Check sheet for the modelled part. Datum: model origin and axes. Units: mm. Face numbers are marked on the shaded views. A direction names the side the tool comes from. Round coordinates to 2 decimals unless told otherwise and drop trailing zeros. Write each loop counter-clockwise with the first axis right and the second up, starting at its lowest first coordinate (ties: lowest second). Pieces come first, ordered by that corner, then holes.
Item 1: Material ranges on line 1 along X through (y, z) = (13, 7.25); line 2 along X through (y, z) = (4.25, 4.5); line 3 along Y through (x, z) = (-0.5, -12), recorded low to high.
Item 2: Section check B-B, the plane x = 8. Record the cut outline in (y, z), plus the area to 3 significant figures.
Item 3: Set-up check for the marked faces 1, 2 and 3: record each of +Z, -Z, +X, -X, +Y, -Y from which the full face is reachable in a straight line by a thin tool's end or side.
Item 4: Section check A-A, the plane z = 0. Record the cut outline in (x, y), plus the area to 3 significant figures.
Item 5: Section check D-D, the plane z = -8. Record the cut outline in (x, y).
Item 6: Depth check by flat-ended pin: pin 1 (1.5 mm diameter, centred on y = 7.5, z = -5.5, fed in from +X); pin 2 (1.6 mm diameter, centred on x = 7.5, z = 0, fed in from +Y); pin 3 (2 mm diameter, centred on x = -13, y = 4, fed in from -Z); pin 4 (3 mm diameter, centred on x = -8, z = 0, fed in from -Y). Enter the tip coordinate at first touch or a pass-through.
Item 7: Release check for a two-part mould opening along Z. For the marked faces 4, 5 and 6 record: pulls with the +Z half, pulls with the -Z half, needs draft (parallel to the pull), parting line crosses it, or undercut.
Item 8: Section check C-C, the plane y = 6.75. Record the cut outline in (x, z).
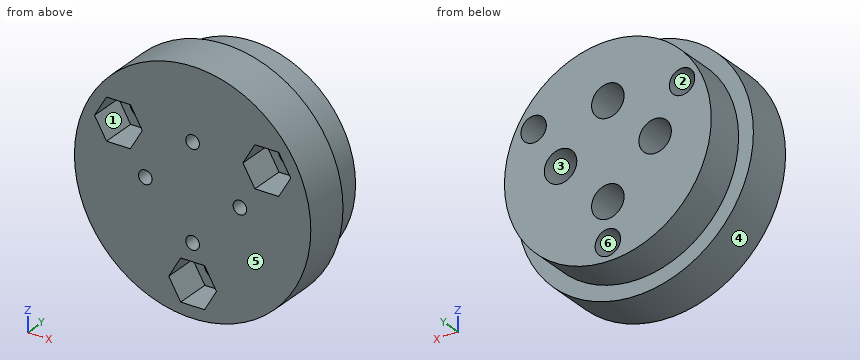
Autodesk Inventor part; units mm, degrees
ref_plane "YZ Plane" through (0, 0, 0) normal (1, 0, 0) x (0, 1, 0)
ref_plane "XZ Plane" through (0, 0, 0) normal (0, 1, 0) x (-1, 0, 0)
ref_plane "XY Plane" through (0, 0, 0) normal (0, 0, 1) x (1, 0, 0)
sketch "Sketch1" plane through (0, 0, 0) normal (0, 1, 0) x (-1, 0, 0)
  circle A0 centre (0, 0) radius 8 construction
  circle A1 centre (8, 0) radius 1 construction
  circle A2 centre (0, -8) radius 1 construction
  circle A3 centre (-8, 0) radius 1 construction
  circle A4 centre (0, 8) radius 1 construction
  circle A5 centre (13, 0) radius 2 construction
  circle A6 centre (-6.5, 11.2583) radius 2 construction
  circle A7 centre (-6.5, -11.2583) radius 2 construction
  line L0 (13, 0) -> (0, 0)
  line L1 (0, 0) -> (0, -5.456)
  circle A8 centre (0, 0) radius 20
  dimension "d0" = 16
  dimension "d1" = 2
  dimension "d2" = 2
  dimension "d3" = 2
  dimension "d4" = 2
  dimension "d5" = 4
  dimension "d8" = 360
  dimension "d10" = 13
  dimension "d11" = 90
  dimension "d12" = 40
extrude "Extrusion1" add sketch "Sketch1" along normal blind 8
sketch "Sketch2" plane through (0, 8, 0) normal (0, 1, 0) x (1, 0, 0)
  circle A0 centre (0, 0) radius 17.5
  dimension "d15" = 35
extrude "Extrusion2" add sketch "Sketch2" along normal blind 6.8
sketch "Sketch3" plane through (0, 14.8, 0) normal (0, 1, 0) x (1, 0, 0)
  circle A0 centre (0, -8) radius 1 construction
  circle A1 centre (-8, 0) radius 1 construction
  circle A2 centre (0, 8) radius 1 construction
  circle A3 centre (8, 0) radius 1 construction
  point P0 (0, 0)
hole "Hole1" at (0, 14.8, -8) at (-8, 14.8, 0) at (0, 14.8, 8) at (8, 14.8, 0) direction (0, -1, 0) diameter 2.3 end through all counterbore diameter 5.5 counterbore depth 6
sketch "Sketch4" plane through (0, 14.8, 0) normal (0, 1, 0) x (1, 0, 0)
  circle A0 centre (0, 0) radius 14.5
  point P0 (0, 14.5)
  point P1 (-12.5574, -7.25)
  point P2 (12.5574, -7.25)
  dimension "d27" = 29
  dimension "d30" = 360
hole "Hole2" at (0, 14.8, -14.5) at (-12.5574, 14.8, 7.25) at (12.5574, 14.8, 7.25) direction (0, -1, 0) diameter 4.3 end through all
sketch "Sketch5" plane through (0, 0, 0) normal (0, -1, 0) x (1, 0, 0)
  circle A0 centre (-12.5574, 7.25) radius 2.15 construction
  circle A1 centre (12.5574, 7.25) radius 2.15 construction
  circle A2 centre (0, -14.5) radius 2.15 construction
  line L0 (4.0415, -14.5) -> (2.0207, -18)
  line L1 (2.0207, -18) -> (-2.0207, -18)
  line L2 (-2.0207, -18) -> (-4.0415, -14.5)
  line L3 (-4.0415, -14.5) -> (-2.0207, -11)
  line L4 (-2.0207, -11) -> (2.0207, -11)
  line L5 (2.0207, -11) -> (4.0415, -14.5)
  line L6 (14.5781, 10.75) -> (16.5988, 7.25)
  line L7 (10.5366, 10.75) -> (14.5781, 10.75)
  line L8 (8.5159, 7.25) -> (10.5366, 10.75)
  line L9 (10.5366, 3.75) -> (8.5159, 7.25)
  line L10 (14.5781, 3.75) -> (10.5366, 3.75)
  line L11 (16.5988, 7.25) -> (14.5781, 3.75)
  line L12 (-16.5988, 7.25) -> (-14.5781, 10.75)
  line L13 (-14.5781, 3.75) -> (-16.5988, 7.25)
  line L14 (-10.5366, 3.75) -> (-14.5781, 3.75)
  line L15 (-8.5159, 7.25) -> (-10.5366, 3.75)
  line L16 (-10.5366, 10.75) -> (-8.5159, 7.25)
  line L17 (-14.5781, 10.75) -> (-10.5366, 10.75)
  point P0 (0, 0)
  dimension "d39" = 7
  dimension "d42" = 360
extrude "Extrusion3" cut sketch "Sketch5" against normal blind 6
properties part number "Arm - slew column A"
Values found:
1. line 1: x = -15.93 to -14.71, -10.41 to -2.65, 2.65 to 10.41, 14.71 to 15.93
1. line 2: x = -19.49 to -15.01, -10.1 to 10.1, 15.01 to 19.49
1. line 3: y = 6 to 14.8
2. outline: (0, -18.33) - (8, -18.33) - (8, -15.56) - (14.8, -15.56) - (14.8, -2.75) - (8.8, -2.75) - (8.8, -1.15) - (0, -1.15) - close; (0, 1.15) - (8.8, 1.15) - (8.8, 2.75) - (14.8, 2.75) - (14.8, 15.56) - (8, 15.56) - (8, 18.33) - (0, 18.33) - close
2. area: 452 mm2
3. face 1: -Y
3. face 2: +Y, -Y
3. face 3: +Y
4. outline: (-20, 0) - (-9.15, 0) - (-9.15, 8.8) - (-10.75, 8.8) - (-10.75, 14.8) - (-17.5, 14.8) - (-17.5, 8) - (-20, 8) - close; (-6.85, 0) - (6.85, 0) - (6.85, 8.8) - (5.25, 8.8) - (5.25, 14.8) - (-5.25, 14.8) - (-5.25, 8.8) - (-6.85, 8.8) - close; (9.15, 0) - (20, 0) - (20, 8) - (17.5, 8) - (17.5, 14.8) - (10.75, 14.8) - (10.75, 8.8) - (9.15, 8.8) - close
4. area: 452 mm2
5. outline: (-18.33, 0) - (-1.15, 0) - (-1.15, 8.8) - (-2.75, 8.8) - (-2.75, 14.8) - (-15.56, 14.8) - (-15.56, 8) - (-18.33, 8) - close; (1.15, 0) - (18.33, 0) - (18.33, 8) - (15.56, 8) - (15.56, 14.8) - (2.75, 14.8) - (2.75, 8.8) - (1.15, 8.8) - close
6. pin 1: stops at x = 19.43
6. pin 2: stops at y = 8.8
6. pin 3: stops at z = -16
6. pin 4: stops at y = 0
7. face 4: parting line crosses it
7. face 5: needs draft
7. face 6: undercut
8. outline: circle Ø40 at (0, 0); hole circle Ø4.3 at (-12.56, 7.25); hole circle Ø2.3 at (-8, 0); hole circle Ø4.3 at (0, -14.5); hole circle Ø2.3 at (0, -8); hole circle Ø2.3 at (0, 8); hole circle Ø2.3 at (8, 0); hole circle Ø4.3 at (12.56, 7.25)
